The listing builds one solid part. Answer for the finished solid, in the listing's coordinates (mm). A direction names the side the tool comes from. Round coordinates to 2 decimals unless told otherwise and drop trailing zeros. Write each loop counter-clockwise with the first axis right and the second up, starting at its lowest first coordinate (ties: lowest second). Pieces come first, ordered by that corner, then holes.
Item 1: For a pull along X with two mould halves and no side action, classify faces 3 (the face through (-1.55, -12.52, -17.81)), 4 (the face through (37.372, -1.449, -2.674)), 5 (the face through (7, -13, 26.435)) as +X half, -X half, draft (parallel to the pull), parting line (faces both ways), or undercut.
Item 2: Find section C-C on z = 4. Give the vertices of the cut face in (x, y).
Item 3: Find section B-B on x = -2. Give the vertices of the cut face in (y, z), then the cut area to 3 significant figures.
Item 4: A tool of negligible diameter and unlimited length cuts with its end or side. For faces 1 (the face through (37.37, -12.59, 24.99)), 2 (the face through (-7.672, -12.522, -10.165)), from which of +Z, -Z, +X, -X, +Y, -Y can it reach the whole face along a straight path? Write none if from no direction.
Item 5: Each of these flat-tipped pins is pushed along its axis until it touches: pin 1 (1.5 mm diameter, centred on y = -22, z = 7.5, fed in from +X); pin 2 (1.5 mm diameter, centred on x = -0.5, y = -21.5, fed in from -Z). Where does it stop, or does it pass through?
Item 6: Find section D-D on x = 35. Give the vertices of the cut face in (y, z), then the cut area to 3 significant figures.
Item 7: Find the intervals of material crossed by probe 1 along X at (y, z) = (-8, 0); probe 2 along Z at (x, y) = (-7, -13.25); probe 3 along X at (y, z) = (-2.5, -12.5), in increasing order.
Item 8: Find section A-A on y = -14.25. Give the vertices of the cut face in (x, z), then the cut area to 3 significant figures.
```python
from build123d import *

# Parameters (mm, degrees)
F0_W         = 63.5255295783
F0_H         = 58.9018370956
F1_DEPTH     = 25.4
F2_R         = 5.08
F3_R         = 5.08
F4_T1_DEPTH  = 15.24
F4_S5_W      = 5.08
F4_S5_H      = 5.08
F4_T6_DEPTH  = 5.08
F4_S11_W     = 5.08
F4_S11_H     = 5.08
F4_T12_DEPTH = 5.08
F4_S17_W     = 5.08
F4_S17_H     = 5.08
F4_T18_DEPTH = 5.08
F4_S23_W     = 5.08
F4_S23_H     = 5.08
F4_T24_DEPTH = 5.08
F4_S29_W     = 5.08
F4_S29_H     = 5.08
F4_T30_DEPTH = 5.08
F4_S35_W     = 5.08
F4_S35_H     = 5.08
F4_T36_DEPTH = 5.08
F4_S41_W     = 5.08
F4_S41_H     = 5.08
F4_T42_DEPTH = 5.08
F4_S47_W     = 5.08
F4_S47_H     = 5.08
F4_T48_DEPTH = 5.08
F6_DEPTH     = 25.401


# Not quite as in the source:
# - a fillet or chamfer that OpenCascade refuses, or shapes differently, is made with other operations: its cross-section is extruded or revolved along the edge and cut away or added


with BuildPart() as f1:
    # F0 (on Front) → F1 (new body)
    with BuildSketch(Plane.XZ):
        with Locations((7.1365712211, -3.0154520646)):
            Rectangle(F0_W, F0_H)
    extrude(amount=F1_DEPTH)

    # F2
    f2_edges = [f1.edges().sort_by_distance(p)[0] for p in [
        (7.136571, -25.4, 26.435466),
        (-24.626194, -25.4, -3.015452),
        (7.136571, -25.4, -32.466371),
        (38.899336, -25.4, -3.015452),
    ]]
    fillet(f2_edges, radius=F2_R)

    # F3
    f3_edges = [f1.edges().sort_by_distance(p)[0] for p in [
        (7.136571, 0, 26.435466),
        (38.899336, 0, -3.015452),
        (-24.626194, 0, -3.015452),
        (7.136571, 0, -32.466371),
    ]]
    fillet(f3_edges, radius=F3_R)

    # F4: fillet of radius 5.08 on 4 edges, made by hand

    # F4_s2 → F4_t1 (cut)
    with BuildSketch(Plane.XZ.offset(5.08)):
        with BuildLine():
            ThreePointArc((33.8193360102, 26.4354664832), (37.4114384586, 24.9475689317), (38.8993360102, 21.3554664832))
            Line((38.8993360102, 21.3554664832), (38.8993360102, 26.4354664832))
            Line((38.8993360102, 26.4354664832), (33.8193360102, 26.4354664832))
        make_face()
        with BuildLine():
            ThreePointArc((38.8993360102, -27.3863706124), (37.4114384586, -30.9784730608), (33.8193360102, -32.4663706124))
            Line((33.8193360102, -32.4663706124), (38.8993360102, -32.4663706124))
            Line((38.8993360102, -32.4663706124), (38.8993360102, -27.3863706124))
        make_face()
        with BuildLine():
            ThreePointArc((-19.5461935681, 26.4354664832), (-23.1382960165, 24.9475689317), (-24.6261935681, 21.3554664832))
            Line((-24.6261935681, 21.3554664832), (-24.6261935681, 26.4354664832))
            Line((-24.6261935681, 26.4354664832), (-19.5461935681, 26.4354664832))
        make_face()
        with BuildLine():
            ThreePointArc((-24.6261935681, -27.3863706124), (-23.1382960165, -30.9784730608), (-19.5461935681, -32.4663706124))
            Line((-19.5461935681, -32.4663706124), (-24.6261935681, -32.4663706124))
            Line((-24.6261935681, -32.4663706124), (-24.6261935681, -27.3863706124))
        make_face()
    extrude(amount=F4_T1_DEPTH, mode=Mode.SUBTRACT)


with BuildPart() as f4_tool4:
    # F4_s5 → F4_t6 (new body)
    with BuildSketch(Plane.YZ.offset(-19.5461935681)):
        with Locations((-2.54, -29.9263706124)):
            Rectangle(F4_S5_W, F4_S5_H)
    extrude(amount=-F4_T6_DEPTH)

    # F4_s7 → F4_t8 (revolve, cut)
    with BuildSketch(Plane(origin=(-19.5461935681, -5.08, -27.3863706124), x_dir=(0, -0.7071067812, 0.7071067812), z_dir=(0, -0.7071067812, -0.7071067812))):
        with BuildLine():
            ThreePointArc((0, -5.08), (5.08, 0), (0, 5.08))
            Line((0, 5.08), (0, -5.08))
        make_face()
    revolve(axis=Axis((-19.5461935681, -5.08, -27.3863706124), (-1, 0, 0)), mode=Mode.SUBTRACT)


with BuildPart() as f1_1:
    add(f1.part)

    # F4_t3: cut F4_tool4
    add(f4_tool4.part, mode=Mode.SUBTRACT)


with BuildPart() as f4_tool10:
    # F4_s11 → F4_t12 (new body)
    with BuildSketch(Plane.YZ.offset(-19.5461935681)):
        with Locations((-22.86, -29.9263706124)):
            Rectangle(F4_S11_W, F4_S11_H)
    extrude(amount=-F4_T12_DEPTH)

    # F4_s13 → F4_t14 (revolve, cut)
    with BuildSketch(Plane(origin=(-19.5461935681, -20.32, -27.3863706124), x_dir=(0, 0.7071067812, 0.7071067812), z_dir=(0, -0.7071067812, 0.7071067812))):
        with BuildLine():
            ThreePointArc((0, -5.08), (5.08, 0), (0, 5.08))
            Line((0, 5.08), (0, -5.08))
        make_face()
    revolve(axis=Axis((-19.5461935681, -20.32, -27.3863706124), (-1, 0, 0)), mode=Mode.SUBTRACT)


with BuildPart() as f1_2:
    add(f1_1.part)

    # F4_t9: cut F4_tool10
    add(f4_tool10.part, mode=Mode.SUBTRACT)


with BuildPart() as f4_tool16:
    # F4_s17 → F4_t18 (new body)
    with BuildSketch(Plane.XY.offset(21.3554664832)):
        with Locations((-22.0861935681, -2.54)):
            Rectangle(F4_S17_W, F4_S17_H)
    extrude(amount=F4_T18_DEPTH)

    # F4_s19 → F4_t20 (revolve, cut)
    with BuildSketch(Plane(origin=(-19.5461935681, -5.08, 21.3554664832), x_dir=(0.7071067812, -0.7071067812, 0), z_dir=(-0.7071067812, -0.7071067812, 0))):
        with BuildLine():
            ThreePointArc((0, -5.08), (5.08, 0), (0, 5.08))
            Line((0, 5.08), (0, -5.08))
        make_face()
    revolve(axis=Axis((-19.5461935681, -5.08, 21.3554664832), (0, 0, 1)), mode=Mode.SUBTRACT)


with BuildPart() as f1_3:
    add(f1_2.part)

    # F4_t15: cut F4_tool16
    add(f4_tool16.part, mode=Mode.SUBTRACT)


with BuildPart() as f4_tool22:
    # F4_s23 → F4_t24 (new body)
    with BuildSketch(Plane.XY.offset(21.3554664832)):
        with Locations((-22.0861935681, -22.86)):
            Rectangle(F4_S23_W, F4_S23_H)
    extrude(amount=F4_T24_DEPTH)

    # F4_s25 → F4_t26 (revolve, cut)
    with BuildSketch(Plane(origin=(-19.5461935681, -20.32, 21.3554664832), x_dir=(0.7071067812, 0.7071067812, 0), z_dir=(0.7071067812, -0.7071067812, 0))):
        with BuildLine():
            ThreePointArc((0, -5.08), (5.08, 0), (0, 5.08))
            Line((0, 5.08), (0, -5.08))
        make_face()
    revolve(axis=Axis((-19.5461935681, -20.32, 21.3554664832), (0, 0, 1)), mode=Mode.SUBTRACT)


with BuildPart() as f1_4:
    add(f1_3.part)

    # F4_t21: cut F4_tool22
    add(f4_tool22.part, mode=Mode.SUBTRACT)


with BuildPart() as f4_tool28:
    # F4_s29 → F4_t30 (new body)
    with BuildSketch(Plane.YZ.offset(33.8193360102)):
        with Locations((-2.54, -29.9263706124)):
            Rectangle(F4_S29_W, F4_S29_H)
    extrude(amount=F4_T30_DEPTH)

    # F4_s31 → F4_t32 (revolve, cut)
    with BuildSketch(Plane(origin=(33.8193360102, -5.08, -27.3863706124), x_dir=(0, -0.7071067812, 0.7071067812), z_dir=(0, 0.7071067812, 0.7071067812))):
        with BuildLine():
            ThreePointArc((0, -5.08), (5.08, 0), (0, 5.08))
            Line((0, 5.08), (0, -5.08))
        make_face()
    revolve(axis=Axis((33.8193360102, -5.08, -27.3863706124), (1, 0, 0)), mode=Mode.SUBTRACT)


with BuildPart() as f1_5:
    add(f1_4.part)

    # F4_t27: cut F4_tool28
    add(f4_tool28.part, mode=Mode.SUBTRACT)


with BuildPart() as f4_tool34:
    # F4_s35 → F4_t36 (new body)
    with BuildSketch(Plane.YZ.offset(33.8193360102)):
        with Locations((-22.86, -29.9263706124)):
            Rectangle(F4_S35_W, F4_S35_H)
    extrude(amount=F4_T36_DEPTH)

    # F4_s37 → F4_t38 (revolve, cut)
    with BuildSketch(Plane(origin=(33.8193360102, -20.32, -27.3863706124), x_dir=(0, 0.7071067812, 0.7071067812), z_dir=(0, 0.7071067812, -0.7071067812))):
        with BuildLine():
            ThreePointArc((0, -5.08), (5.08, 0), (0, 5.08))
            Line((0, 5.08), (0, -5.08))
        make_face()
    revolve(axis=Axis((33.8193360102, -20.32, -27.3863706124), (1, 0, 0)), mode=Mode.SUBTRACT)


with BuildPart() as f1_6:
    add(f1_5.part)

    # F4_t33: cut F4_tool34
    add(f4_tool34.part, mode=Mode.SUBTRACT)


with BuildPart() as f4_tool40:
    # F4_s41 → F4_t42 (new body)
    with BuildSketch(Plane.XY.offset(21.3554664832)):
        with Locations((36.3593360102, -2.54)):
            Rectangle(F4_S41_W, F4_S41_H)
    extrude(amount=F4_T42_DEPTH)

    # F4_s43 → F4_t44 (revolve, cut)
    with BuildSketch(Plane(origin=(33.8193360102, -5.08, 21.3554664832), x_dir=(-0.7071067812, -0.7071067812, 0), z_dir=(-0.7071067812, 0.7071067812, 0))):
        with BuildLine():
            ThreePointArc((0, -5.08), (5.08, 0), (0, 5.08))
            Line((0, 5.08), (0, -5.08))
        make_face()
    revolve(axis=Axis((33.8193360102, -5.08, 21.3554664832), (0, 0, 1)), mode=Mode.SUBTRACT)


with BuildPart() as f1_7:
    add(f1_6.part)

    # F4_t39: cut F4_tool40
    add(f4_tool40.part, mode=Mode.SUBTRACT)


with BuildPart() as f4_tool46:
    # F4_s47 → F4_t48 (new body)
    with BuildSketch(Plane.XY.offset(21.3554664832)):
        with Locations((36.3593360102, -22.86)):
            Rectangle(F4_S47_W, F4_S47_H)
    extrude(amount=F4_T48_DEPTH)

    # F4_s49 → F4_t50 (revolve, cut)
    with BuildSketch(Plane(origin=(33.8193360102, -20.32, 21.3554664832), x_dir=(-0.7071067812, 0.7071067812, 0), z_dir=(0.7071067812, 0.7071067812, 0))):
        with BuildLine():
            ThreePointArc((0, -5.08), (5.08, 0), (0, 5.08))
            Line((0, 5.08), (0, -5.08))
        make_face()
    revolve(axis=Axis((33.8193360102, -20.32, 21.3554664832), (0, 0, 1)), mode=Mode.SUBTRACT)


with BuildPart() as f1_8:
    add(f1_7.part)

    # F4_t45: cut F4_tool46
    add(f4_tool46.part, mode=Mode.SUBTRACT)

    # F5 (on face) → F6 (cut, through all)
    with BuildSketch(Plane(origin=(0, 0, 0), x_dir=(-1, 0, 0), z_dir=(0, 1, 0))):
        with BuildLine():
            ThreePointArc((6.7243616166, -9.373779083), (8.3427349026, -4.8105260449), (8.8915969563, 0))
            ThreePointArc((8.8915969563, 0), (-31.6040146397, 9.4715782097), (0.4899266998, -16.978077395))
            ThreePointArc((0.4899266998, -16.978077395), (0.2228411144, -10.4012847151), (6.7243616166, -9.373779083))
        make_face()
        with BuildLine():
            ThreePointArc((6.7243616166, -9.373779083), (0.2228411144, -10.4012847151), (0.4899266998, -16.978077395))
            ThreePointArc((0.4899266998, -16.978077395), (4.0507851492, -13.5396502777), (6.7243616166, -9.373779083))
        make_face()
        with BuildLine():
            ThreePointArc((6.7243616166, -9.373779083), (4.0507851492, -13.5396502777), (0.4899266998, -16.978077395))
            ThreePointArc((0.4899266998, -16.978077395), (1.5703386286, -17.823326152), (2.8412431673, -18.3395984162))
            ThreePointArc((2.8412431673, -18.3395984162), (4.5469228112, -13.9210498797), (8.3783969439, -11.136679181))
            ThreePointArc((8.3783969439, -11.136679181), (7.6606485066, -10.152707633), (6.7243616166, -9.373779083))
        make_face()
        with BuildLine():
            ThreePointArc((9.0007845368, -13.5396502777), (7.0934206735, -17.4441173353), (2.8412431673, -18.3395984162))
            ThreePointArc((2.8412431673, -18.3395984162), (10.8393587072, -27.3794387001), (19.5461935681, -19.0200373308))
            ThreePointArc((19.5461935681, -19.0200373308), (16.0046689137, -12.1850717648), (8.3783969439, -11.136679181))
            ThreePointArc((8.3783969439, -11.136679181), (8.842662113, -12.2985180922), (9.0007845368, -13.5396502777))
        make_face()
        with BuildLine():
            ThreePointArc((8.3783969439, -11.136679181), (4.5469228112, -13.9210498797), (2.8412431673, -18.3395984162))
            ThreePointArc((2.8412431673, -18.3395984162), (7.0934206735, -17.4441173353), (9.0007845368, -13.5396502777))
            ThreePointArc((9.0007845368, -13.5396502777), (8.842662113, -12.2985180922), (8.3783969439, -11.136679181))
        make_face()
    extrude(amount=-F6_DEPTH, mode=Mode.SUBTRACT)


solid = f1_8.part
```
Check values:
1. face 3: undercut
1. face 4: +X half
1. face 5: draft
2. outline: (-24.63, -20.32) arc R5.08 ccw to (-19.55, -25.4) - (-8.51, -25.4) - (-8.51, 0) - (-19.55, 0) arc R5.08 ccw to (-24.63, -5.08) - close; (33.44, -25.4) - (33.82, -25.4) arc R5.08 ccw to (38.9, -20.32) - (38.9, -5.08) arc R5.08 ccw to (33.82, 0) - (33.44, 0) - close
3. outline: (-25.4, -27.39) arc R5.08 ccw to (-20.32, -32.47) - (-5.08, -32.47) arc R5.08 ccw to (0, -27.39) - (0, -18.04) - (-25.4, -18.04) - close; (-25.4, 15.71) - (0, 15.71) - (0, 21.36) arc R5.08 ccw to (-5.08, 26.44) - (-20.32, 26.44) arc R5.08 ccw to (-25.4, 21.36) - close
3. area: 617 mm2
4. face 1: +Z, +X, +Y, -Y
4. face 2: +Y, -Y
5. pin 1: stops at x = 38.81
5. pin 2: stops at z = -32.45
6. outline: (-25.26, -27.39) arc R4.94 ccw to (-20.32, -32.33) - (-5.08, -32.33) arc R4.94 ccw to (-0.14, -27.39) - (-0.14, 21.36) arc R4.94 ccw to (-5.08, 26.3) - (-20.32, 26.3) arc R4.94 ccw to (-25.26, 21.36) - close
6. area: 1,450 mm2
7. probe 1: x = -24.63 to -8.89, 33.82 to 38.9
7. probe 2: z = -32.47 to -26.27, -9.56 to -8.79, 8.79 to 26.44
7. probe 3: x = -23.92 to -16.42, 29.78 to 38.2
8. outline: (-24.63, -27.39) arc R5.08 ccw to (-19.55, -32.47) - (33.82, -32.47) arc R5.08 ccw to (38.9, -27.39) - (38.9, 21.36) arc R5.08 ccw to (33.82, 26.44) - (-19.55, 26.44) arc R5.08 ccw to (-24.63, 21.36) - close; hole (-8.38, -11.14) arc R8.37 ccw (long way) to (-2.84, -18.34) arc R4.95 ccw to (-0.49, -16.98) arc R21.36 ccw (long way) to (-6.72, -9.37) arc R4.95 ccw to start
8. area: 2,050 mm2
